Verification items for the finished model (mm, model axes). A direction names the side the tool comes from. Give positions to 0.01 mm unless a question says otherwise; leave off trailing zeros. Loops run counter-clockwise (first coordinate to the right, second up) from the corner with the lowest first, then second, coordinate; pieces in that order, holes last. Notation, with made-up numbers: (38, -29) - (59, -29) arc R19 ccw to (59, -24) - close; hole circle Ø7 at (-30.5, -14.75). An arc over 180 degrees is marked (long way). One line per item, written item: value. Start each with the question number.
1. Sectioned sample at A-A (z = -4.5). Record the cut outline in (x, y), plus the area to 3 significant figures.
2. Sectioned sample at B-B (z = 46). Record the cut outline in (x, y), plus the area to 3 significant figures.
3. Gauge pin test, flat ends, axial feed: pin 1 (5 mm diameter, centred on x = -66, z = -44, fed in from +Y); pin 2 (16.5 mm diameter, centred on y = 51.5, z = -3.5, fed in from +X); pin 3 (1.4 mm diameter, centred on x = 64.5, y = 37.5, fed in from -Z). Record the tip position at first contact, or that the pin passes through.
4. Access from +Z, -Z, +X, -X, +Y, -Y to the whole of each face (thin tool, end or side, straight path). Record for faces 4 (the flat face through (60, 41, -42.5)), 5 (the flat face through (-42.5, 12, -46)), 6 (the flat face through (-35, 64, 29.5)), 7 (the flat face through (35, 74, -31)), 8 (the flat face through (-64, 41, -39.5)).
5. Mould release check, pull along X, two halves, no side actions. Record for faces 1 (the flat face through (58.342, 41, -46)), 2 (the flat face through (64, 12, 28)), 3 (the flat face through (-40, 60, -32)): pulls with the +X half, pulls with the -X half, needs draft (parallel to the pull), parting line crosses it, or undercut.
6. Sectioned sample at D-D (y = 63). Count the separate pieces of the cut face and the enclosed holes in it, plus the area to 3 significant figures.
7. Sectioned sample at C-C (x = 45). Record the cut outline in (y, z), plus the area to 3 significant figures.
8. Scan lines: L1, parallel to X at y = 76, z = 46; L2, parallel to X at y = 2.8, z = 46; L3, parallel to X at y = 70, z = -41.5. Record each from-to range of solid material in increasing order. Write a range as [from, to].
from build123d import *

# Parameters (mm, degrees)
BOSS_EXTRUDE1_DEPTH     = 4
CUT_EXTRUDE3_REACH      = 86.48
SKETCH3_R               = 1.6
SKETCH4_W               = 116.684034766
SKETCH4_H               = 7
BOSS_EXTRUDE2_DEPTH     = 75
SKETCH1_3_W             = 5
SKETCH1_3_H             = 5
BOSS_EXTRUDE3_DEPTH     = 79
SKETCH5_W               = 85
SKETCH5_H               = 25
CUT_EXTRUDE4_DEPTH      = 144.918835946
CUT_EXTRUDE5_DEPTH      = 166.450220187
CUT_EXTRUDE5_DEPTH_BACK = 166.450220187
SKETCH6_W               = 56
SKETCH6_H               = 25
SKETCH7_R               = 2.2
CUT_EXTRUDE6_DEPTH      = 10
SKETCH8_W               = 10
SKETCH8_H               = 4
BOSS_EXTRUDE4_DEPTH     = 13
SKETCH9_W               = 10
SKETCH9_H               = 3
BOSS_EXTRUDE5_DEPTH     = 15
FILLET1_R               = 5
MIRROR2_COPY_1_SKETCH_W = 10
MIRROR2_COPY_1_SKETCH_H = 4
MIRROR2_COPY_1_DEPTH    = 13
MIRROR2_COPY_2_SKETCH_W = 10
MIRROR2_COPY_2_SKETCH_H = 3
MIRROR2_COPY_2_DEPTH    = 15


with BuildPart() as part:
    # Sketch1 → Boss-Extrude1 (new body)
    # profile 1 of 3: a face of its own
    with BuildSketch(Plane(origin=(0, 0, 0), x_dir=(1, 0, 0), z_dir=(0, 1, 0))):
        Polygon((-68.342017383, -9.5), (-68.342017383, -49.5), (68.342017383, -49.5), (68.342017383, -9.5), (63.842017383, -9.5), (63.842017383, 9.5), (68.342017383, 9.5), (68.342017383, 49.5), (-68.342017383, 49.5), (-68.342017383, 9.5), (-63.842017383, 9.5), (-63.842017383, -9.5), align=None)
        Polygon((-56.342017383, -42.5), (-61.342017383, -42.5), (-61.342017383, -37.5), (-61.342017383, 37.5), (-61.342017383, 42.5), (-56.342017383, 42.5), (56.342017383, 42.5), (61.342017383, 42.5), (61.342017383, 37.5), (61.342017383, -37.5), (61.342017383, -42.5), (56.342017383, -42.5), align=None, mode=Mode.SUBTRACT)
    # profile 2 of 3: a face of its own
    with BuildSketch(Plane(origin=(0, 0, 0), x_dir=(1, 0, 0), z_dir=(0, 1, 0))):
        Polygon((-68.342017383, -7.5), (-68.342017383, -9.5), (-63.842017383, -9.5), (-63.842017383, 9.5), (-68.342017383, 9.5), (-68.342017383, 7.5), (-65.842017383, 7.5), (-65.842017383, -7.5), align=None)
    # profile 3 of 3: a face of its own
    with BuildSketch(Plane(origin=(0, 0, 0), x_dir=(1, 0, 0), z_dir=(0, 1, 0))):
        Polygon((63.842017383, -9.5), (68.342017383, -9.5), (68.342017383, -7.5), (65.842017383, -7.5), (65.842017383, 7.5), (68.342017383, 7.5), (68.342017383, 9.5), (63.842017383, 9.5), align=None)
    extrude(amount=BOSS_EXTRUDE1_DEPTH)

    # Sketch3 → Cut-Extrude3 (cut, up to next)
    with BuildSketch(Plane(origin=(0, 0, 0), x_dir=(1, 0, 0), z_dir=(0, 1, 0)), mode=Mode.PRIVATE) as cut_extrude3_sk1:
        with Locations(Location((-64.842017383, 46, 0), (0, 0, 270))):
            Circle(SKETCH3_R)
    cut_extrude3_tool1 = extrude(cut_extrude3_sk1.sketch, amount=CUT_EXTRUDE3_REACH, mode=Mode.PRIVATE) & part.part
    # Sketch3 → Cut-Extrude3 (cut, up to next)
    with BuildSketch(Plane(origin=(0, 0, 0), x_dir=(1, 0, 0), z_dir=(0, 1, 0)), mode=Mode.PRIVATE) as cut_extrude3_sk2:
        with Locations(Location((-64.842017383, -46, 0), (0, 0, 270))):
            Circle(SKETCH3_R)
    cut_extrude3_tool2 = extrude(cut_extrude3_sk2.sketch, amount=CUT_EXTRUDE3_REACH, mode=Mode.PRIVATE) & part.part
    # Sketch3 → Cut-Extrude3 (cut, up to next)
    with BuildSketch(Plane(origin=(0, 0, 0), x_dir=(1, 0, 0), z_dir=(0, 1, 0)), mode=Mode.PRIVATE) as cut_extrude3_sk3:
        with Locations(Location((64.842017383, -46, 0), (0, 0, 270))):
            Circle(SKETCH3_R)
    cut_extrude3_tool3 = extrude(cut_extrude3_sk3.sketch, amount=CUT_EXTRUDE3_REACH, mode=Mode.PRIVATE) & part.part
    # Sketch3 → Cut-Extrude3 (cut, up to next)
    with BuildSketch(Plane(origin=(0, 0, 0), x_dir=(1, 0, 0), z_dir=(0, 1, 0)), mode=Mode.PRIVATE) as cut_extrude3_sk4:
        with Locations(Location((64.842017383, 46, 0), (0, 0, 270))):
            Circle(SKETCH3_R)
    cut_extrude3_tool4 = extrude(cut_extrude3_sk4.sketch, amount=CUT_EXTRUDE3_REACH, mode=Mode.PRIVATE) & part.part
    add(cut_extrude3_tool1.solids().sort_by_distance((-64.842017, 0, -46))[0], mode=Mode.SUBTRACT)
    add(cut_extrude3_tool2.solids().sort_by_distance((-64.842017, 0, 46))[0], mode=Mode.SUBTRACT)
    add(cut_extrude3_tool3.solids().sort_by_distance((64.842017, 0, 46))[0], mode=Mode.SUBTRACT)
    add(cut_extrude3_tool4.solids().sort_by_distance((64.842017, 0, -46))[0], mode=Mode.SUBTRACT)

    # Sketch4 → Boss-Extrude2 (add)
    with BuildSketch(Plane(origin=(0, 4, 0), x_dir=(1, 0, 0), z_dir=(0, 1, 0))):
        Polygon((-61.342017383, -39.5), (-61.342017383, 39.5), (-65.904231228, 39.5), (-65.904231228, 7.5), (-65.842017383, 7.5), (-65.842017383, -7.5), (-65.904231228, -7.5), (-65.904231228, -39.5), align=None)
        with Locations((0, 46)):
            Rectangle(SKETCH4_W, SKETCH4_H)
        with Locations((0, -46)):
            Rectangle(SKETCH4_W, SKETCH4_H)
        Polygon((65.904231228, 39.5), (61.342017383, 39.5), (61.342017383, -39.5), (65.904231228, -39.5), (65.904231228, -7.5), (65.842017383, -7.5), (65.842017383, 7.5), (65.904231228, 7.5), align=None)
    extrude(amount=BOSS_EXTRUDE2_DEPTH)

    # Sketch1_3 → Boss-Extrude3 (add)
    with BuildSketch(Plane(origin=(0, 0, 0), x_dir=(1, 0, 0), z_dir=(0, 1, 0))):
        with Locations((-58.842017383, 40)):
            Rectangle(SKETCH1_3_W, SKETCH1_3_H)
        with Locations((-58.842017383, -40)):
            Rectangle(SKETCH1_3_W, SKETCH1_3_H)
        with Locations((58.842017383, -40)):
            Rectangle(SKETCH1_3_W, SKETCH1_3_H)
        with Locations((58.842017383, 40)):
            Rectangle(SKETCH1_3_W, SKETCH1_3_H)
    extrude(amount=BOSS_EXTRUDE3_DEPTH)

    # Sketch5 → Cut-Extrude4 (cut, through all)
    with BuildSketch(Plane.XY.offset(49.5)):
        with Locations((0, 12.5)):
            Rectangle(SKETCH5_W, SKETCH5_H)
    extrude(amount=-CUT_EXTRUDE4_DEPTH, mode=Mode.SUBTRACT)

    # Sketch6 → Cut-Extrude5 (cut, two sides: drawn at the far end of the back side and taken through both)
    with BuildSketch(Plane(origin=(68.342017383, 0, 0), x_dir=(0, 0, -1), z_dir=(1, 0, 0)).offset(-CUT_EXTRUDE5_DEPTH_BACK)):
        with Locations((0, 12.5)):
            Rectangle(SKETCH6_W, SKETCH6_H)
    extrude(amount=CUT_EXTRUDE5_DEPTH + CUT_EXTRUDE5_DEPTH_BACK, mode=Mode.SUBTRACT)

    # Sketch7 → Cut-Extrude6 (cut)
    with BuildSketch(Plane(origin=(0, 79, 0), x_dir=(1, 0, 0), z_dir=(0, 1, 0))):
        with Locations(Location((40.521857066, 46, 0), (0, 0, 270))):
            Circle(SKETCH7_R)
        with Locations(Location((-39.478142934, 46, 0), (0, 0, 270))):
            Circle(SKETCH7_R)
        with Locations(Location((40.521857066, -46, 0), (0, 0, 270))):
            Circle(SKETCH7_R)
        with Locations(Location((-39.478142934, -46, 0), (0, 0, 270))):
            Circle(SKETCH7_R)
    extrude(amount=-CUT_EXTRUDE6_DEPTH, mode=Mode.SUBTRACT)

    # Sketch8 → Boss-Extrude4 (add)
    with BuildSketch(Plane.XY.offset(-42.5)):
        with Locations((-35, 57)):
            Rectangle(SKETCH8_W, SKETCH8_H)
    boss_extrude4 = extrude(amount=BOSS_EXTRUDE4_DEPTH)

    # Sketch9 → Boss-Extrude5 (add)
    with BuildSketch(Plane(origin=(0, 59, 0), x_dir=(1, 0, 0), z_dir=(0, 1, 0))):
        with Locations((-35, 31)):
            Rectangle(SKETCH9_W, SKETCH9_H)
    boss_extrude5 = extrude(amount=BOSS_EXTRUDE5_DEPTH)

    # Fillet1
    fillet1_edges = [part.edges().sort_by_distance(p)[0] for p in [
        (-35, 55, -42.5),
    ]]
    fillet(fillet1_edges, radius=FILLET1_R)

    # Mirror1: Boss-Extrude4, Boss-Extrude5 across plane
    add(boss_extrude4.mirror(Plane.XY))
    add(boss_extrude5.mirror(Plane.XY))

    # Mirror2: Boss-Extrude4, Boss-Extrude5 across plane
    add(boss_extrude4.mirror(Plane(origin=(0, 0, 0), x_dir=(0, 0, 1), z_dir=(1, 0, 0))))
    add(boss_extrude5.mirror(Plane(origin=(0, 0, 0), x_dir=(0, 0, 1), z_dir=(1, 0, 0))))

    # Mirror2 copy 1 sketch → Mirror2 copy 1 (add)
    with BuildSketch(Plane(origin=(0, 0, 42.5), x_dir=(-1, 0, 0), z_dir=(0, 0, -1))):
        with Locations((-35, 57)):
            Rectangle(MIRROR2_COPY_1_SKETCH_W, MIRROR2_COPY_1_SKETCH_H)
    extrude(amount=MIRROR2_COPY_1_DEPTH)

    # Mirror2 copy 2 sketch → Mirror2 copy 2 (add)
    with BuildSketch(Plane(origin=(0, 59, 0), x_dir=(-1, 0, 0), z_dir=(0, 1, 0))):
        with Locations((-35, 31)):
            Rectangle(MIRROR2_COPY_2_SKETCH_W, MIRROR2_COPY_2_SKETCH_H)
    extrude(amount=MIRROR2_COPY_2_DEPTH)


solid = part.part
Results are:
1. outline: (-65.84, 25) - (-61.34, 25) - (-61.34, 79) - (-65.84, 79) - close; (61.34, 25) - (65.84, 25) - (65.84, 79) - (61.34, 79) - close
1. area: 486 mm^2
2. outline: (-68.34, 0) - (-66.44, 0) - (-66.44, 4) - (-68.34, 4) - close; (-63.24, 0) - (-42.5, 0) - (-42.5, 25) - (42.5, 25) - (42.5, 0) - (63.24, 0) - (63.24, 4) - (58.34, 4) - (58.34, 79) - (42.72, 79) - (42.72, 69) - (38.32, 69) - (38.32, 79) - (-37.28, 79) - (-37.28, 69) - (-41.68, 69) - (-41.68, 79) - (-58.34, 79) - (-58.34, 4) - (-63.24, 4) - close; (66.44, 0) - (68.34, 0) - (68.34, 4) - (66.44, 4) - close
2. area: 7,060 mm^2
3. pin 1: stops at y = 4
3. pin 2: stops at x = 65.9
3. pin 3: stops at z = -39.5
4. face 4: -Z, +X, +Y
4. face 5: +Z, -Z, -Y
4. face 6: +Y, -Y
4. face 7: +Y
4. face 8: -Z, -X, +Y
5. face 1: pulls with the +X half
5. face 2: needs draft
5. face 3: undercut
6. separate pieces: 5
6. enclosed holes: 1
6. area: 2,570 mm^2
7. outline: (0, -49.5) - (79, -49.5) - (79, -42.5) - (0, -42.5) - close; (0, 42.5) - (79, 42.5) - (79, 49.5) - (0, 49.5) - close
7. area: 1,110 mm^2
8. L1: x = [-58.34, -41.68], [-37.28, 38.32], [42.72, 58.34]
8. L2: x = [-68.34, -66.44], [-63.24, -42.5], [42.5, 63.24], [66.44, 68.34]
8. L3: x = [-61.34, -56.34], [56.34, 61.34]
